from build123d import *

# Parameters (mm, degrees)
BOSS_EXTRUDE1_DEPTH = 6.35
SKETCH3_R           = 1.5621
CUT_EXTRUDE1_DEPTH  = 7.35


with BuildPart() as part:
    # Sketch1 → Boss-Extrude1 (new body)
    with BuildSketch(Plane(origin=(0, 0, 0), x_dir=(1, 0, 0), z_dir=(0, 1, 0))):
        with BuildLine():
            Line((-63.5, 59.072409794), (-63.5, 20.592039538))
            ThreePointArc((-63.5, 20.592039538), (-33.377694994, 5.276670816), (0, 0))
            Line((0, 0), (0, 76.2))
            ThreePointArc((0, 76.2), (-16.843183971, 80.990709686), (-28.643822974, 93.92858682))
            Line((-28.643822974, 93.92858682), (-63.5, 59.072409794))
        make_face()
    boss_extrude1 = extrude(amount=BOSS_EXTRUDE1_DEPTH)

    # Mirror1: Boss-Extrude1 across plane
    add(boss_extrude1.mirror(Plane(origin=(0, 0, 0), x_dir=(0, 0, 1), z_dir=(1, 0, 0))))

    # Sketch3 → Cut-Extrude1 (cut, through all)
    with BuildSketch(Plane(origin=(0, 6.35, 0), x_dir=(1, 0, 0), z_dir=(0, 1, 0))):
        with Locations((-41.3131, 19.05)):
            Circle(SKETCH3_R)
        with Locations((41.3131, 19.05)):
            Circle(SKETCH3_R)
        with Locations((-41.3131, 67.3862)):
            Circle(SKETCH3_R)
        with Locations((33.8201, 67.3862)):
            Circle(SKETCH3_R)
    extrude(amount=-CUT_EXTRUDE1_DEPTH, mode=Mode.SUBTRACT)


solid = part.part
The listing builds one solid part. Answer for the finished solid, in the listing's coordinates (mm). Give positions to 0.01 mm unless a question says otherwise; leave off trailing zeros. Loops run counter-clockwise (first coordinate to the right, second up) from the corner with the lowest first, then second, coordinate; pieces in that order, holes last. Notation, with made-up numbers: (86.25, 56) - (122.25, 56) arc R34 ccw to (122.25, 86) - close; hole circle Ø6 at (-10.75, 57.5). An arc over 180 degrees is marked (long way). Use one line per item in the form item = value.
1. Section B-B on y = 1.5 is taken. Give the vertices of the cut face in (x, z), then the cut area to 3 significant figures.
Calculated:
outline = (-63.5, -59.07) - (-28.64, -93.93) arc R32 cw to (28.64, -93.93) - (63.5, -59.07) - (63.5, -20.59) arc R108.2 ccw to (-63.5, -20.59) - close; hole circle Ø3.12 at (-41.31, -67.39); hole circle Ø3.12 at (-41.31, -19.05); hole circle Ø3.12 at (33.82, -67.39); hole circle Ø3.12 at (41.31, -19.05)
area = 9,120 mm^2
2. Given pin 1 Ø1.5 at (x, y) = (-33, 4) entering from -Z; pin 2 Ø4 at (x, z) = (41.31, -19.05) entering from -Y; pin 3 Ø2 at (x, y) = (-35, 4.5) entering from +Z; pin 4 Ø2.5 at (x, z) = (33.82, -67.39) entering from +Y, each flat-ended and moving along its own axis, determine where each tip first touches the part or whether it passes through.
Calculated:
pin_1 = -90.32
pin_2 = 0
pin_3 = -5.48
pin_4 = through
3. The mould has two halves that part along X. Classify faces 1 (the face through (40.162, 3.219, -20.106)), 2 (the face through (1, 6.35, -48)), 3 (the face through (63.5, 3, -40)): pulls with the +X half, pulls with the -X half, needs draft (parallel to the pull), parting line crosses it, or undercut.
Calculated:
face_1 = undercut
face_2 = needs draft
face_3 = pulls with the +X half
4. Section A-A on z = -19.05 is taken. Give the vertices of the cut face in (x, y), then the cut area to 3 significant figures.
Calculated:
outline = (-61.32, 0) - (-42.88, 0) - (-42.88, 6.35) - (-61.32, 6.35) - close; (-39.75, 0) - (39.75, 0) - (39.75, 6.35) - (-39.75, 6.35) - close; (42.88, 0) - (61.32, 0) - (61.32, 6.35) - (42.88, 6.35) - close
area = 739 mm^2
5. Section C-C on x = 17 is taken. Give the vertices of the cut face in (y, z).
Calculated:
outline = (0, -81.09) - (6.35, -81.09) - (6.35, -1.34) - (0, -1.34) - close
6. Find the intervals of material crossed by line 1 along X through (y, z) = (3, -19.05); line 2 along X through (y, z) = (1, -83); line 3 along X through (y, z) = (2.25, -71), in increasing order. Write a range as [from, to].
Calculated:
line_1 = [-61.32, -42.88], [-39.75, 39.75], [42.88, 61.32]
line_2 = [-39.57, -19.72], [19.72, 39.57]
line_3 = [-51.57, 51.57]
7. Section D-D on x = -14.5 is taken. Give the vertices of the cut face in (y, z), then the cut area to 3 significant figures.
Calculated:
outline = (0, -79.67) - (6.35, -79.67) - (6.35, -0.98) - (0, -0.98) - close
area = 500 mm^2
